```python
from build123d import *

# Parameters (mm, degrees)
F0_R     = 26.3604411939
F1_DEPTH = 100.000054
F3_R     = 1.999996
F4_DEPTH = 76.2


with BuildPart() as f1:
    # F0 (on Top) → F1 (new body)
    with BuildSketch(Plane.XY):
        Circle(F0_R)
    extrude(amount=F1_DEPTH)


with BuildPart() as f4:
    # F3 (on Top) → F4 (new body)
    with BuildSketch(Plane.XY):
        Circle(F3_R)
    extrude(amount=F4_DEPTH)


solid = f4.part
```
CAD build for the part. Positions are in the model's coordinates, mm. Give positions to 0.01 mm unless a question says otherwise; leave off trailing zeros. Loops run counter-clockwise (first coordinate to the right, second up) from the corner with the lowest first, then second, coordinate; pieces in that order, holes last. Notation, with made-up numbers: (-2.75, -24) -> (40.25, -24) arc R13 ccw to (40.25, 1) -> close; hole circle Ø7 at (47.5, -25). An arc over 180 degrees is marked (long way). Use a Markdown table: item, result.
1. Flat gauge pins, fed straight in: pin 1 (1.5 mm diameter, centred on x = -1, z = 14, fed in from +Y); pin 2 (1.5 mm diameter, centred on y = 1, z = 17, fed in from -X). Where does each tip first touch, or does it go through?
Check result:
| item | result |
|---|---|
| pin 1 | stops at y = 1.98 |
| pin 2 | stops at x = -1.98 |
2. Slice it at C-C (y = -0.95). List the corners of the cut face in (x, z), plus the area to 3 significant figures.
Check result:
| item | result |
|---|---|
| outline | (-1.76, 0) -> (1.76, 0) -> (1.76, 76.2) -> (-1.76, 76.2) -> close |
| area | 268 mm^2 |
3. Wall check: L1, parallel to Y at x = -0.35, z = 20.5; L2, parallel to X at y = 0.9, z = 12.5; L3, parallel to X at y = 0.4, z = 45.5. Give the ranges that are in metal, low to high. Write a range as [from, to].
Check result:
| item | result |
|---|---|
| L1 | y = [-1.97, 1.97] |
| L2 | x = [-1.79, 1.79] |
| L3 | x = [-1.96, 1.96] |
4. Slice it at B-B (x = -0.6). List the corners of the cut face in (y, z).
Check result:
| item | result |
|---|---|
| outline | (-1.91, 0) -> (1.91, 0) -> (1.91, 76.2) -> (-1.91, 76.2) -> close |
5. Slice it at A-A (z = 35.5). List the corners of the cut face in (x, y).
Check result:
| item | result |
|---|---|
| outline | circle Ø4 at (0, 0) |
